Can you work these out from the model? Positions are in its coordinate system, mm. Face numbers are marked on the shaded views. A direction names the side the tool comes from. Coordinates: 2 decimals unless noted, no trailing zeros. Order: outer loops, then holes, each group sorted by start corner. A loop starts at its lowest first (then second) coordinate and runs counter-clockwise, first axis right, second up. Notation, with made-up numbers: (79, 78) -> (94, 78) arc R31 cw to (94, 106) -> close; hole circle Ø2 at (-14, 52). An arc over 180 degrees is marked (long way). Return JSON: item names as keys, results as strings. Group by question number.
1) If I drill on probe 1 along Z at (x, y) = (0, -1); probe 2 along X at (y, z) = (0.75, 209.55); probe 3 along X at (y, z) = (-2, 209.55), over which ranges is the centre line in solid material (lowest first)? Write a range as from..to.
2) For pin 1 (5 mm diameter, centred on x = -0.5, z = 205, fed in from -Y); pin 2 (3 mm diameter, centred on x = -1, z = 211, fed in from -Y); pin 3 (5 mm diameter, centred on x = -18.5, y = -16, fed in from +Z); pin 4 (2 mm diameter, centred on x = -44.5, y = -47.5, fed in from -Z), each with a flat end and sliding along its axis, tell me the tip position at first contact or that it passes through.
3) If we section it at A-A, the plane z = 161.5: Please give me the cut outline in (x, y), then the cut area to 3 significant figures.
4) For the marked faces 1 and 2, which set-ups out of +Z, -Z, +X, -X, +Y, -Y let a thin tool reach every point of the face, with its end or its side?
from build123d import *

# Parameters (mm, degrees)
F0_R      = 69.85
F1_DEPTH  = 12.7
F4_R      = 5.08
F5_R      = 6.35
F6_DEPTH  = 203.2
F8_DEPTH  = 12.7
F9_R      = 3.81
F10_DEPTH = 12.7
F11_R     = 5.08


with BuildPart() as f1:
    # F0 (on Top) → F1 (new body)
    with BuildSketch(Plane.XY):
        Circle(F0_R)
    extrude(amount=F1_DEPTH)

    # F2 (on Front) → F3 (revolve)
    with BuildSketch(Plane.XZ):
        Polygon((0, 50.8), (-69.85, 12.7), (0, 12.7), align=None)
    revolve(axis=Axis((0, 0, 31.75), (0, 0, -1)))

    # F4
    f4_edges = [f1.edges().sort_by_distance(p)[0] for p in [
        (0, -69.85, 12.7),
        (0, 69.85, 12.7),
    ]]
    fillet(f4_edges, radius=F4_R)

    # F5 (on Top) → F6 (join)
    with BuildSketch(Plane.XY):
        Circle(F5_R)
    extrude(amount=F6_DEPTH)

    # F7 (on face) → F8 (join)
    with BuildSketch(Plane.XY.offset(203.2)):
        with BuildLine():
            ThreePointArc((-3.81, 5.08), (-6.35, 0), (-3.81, -5.08))
            Line((-3.81, -5.08), (3.81, -5.08))
            ThreePointArc((3.81, -5.08), (6.35, 0), (3.81, 5.08))
            Line((3.81, 5.08), (-3.81, 5.08))
        make_face()
    extrude(amount=F8_DEPTH)

    # F9 (on face) → F10 (cut, symmetric)
    with BuildSketch(Plane.XZ.offset(5.08)):
        with Locations((0, 209.55)):
            Circle(F9_R)
    extrude(amount=F10_DEPTH, both=True, mode=Mode.SUBTRACT)

    # F11
    f11_edges = [f1.edges().sort_by_distance(p)[0] for p in [
        (0, -6.35, 47.336364),
        (0, 6.35, 47.336364),
        (-36.776284, 0, 30.740209),
        (3.3e-05, 67.202608, 14.144033),
        (3.3e-05, -67.202608, 14.144033),
    ]]
    fillet(f11_edges, radius=F11_R)


solid = f1.part
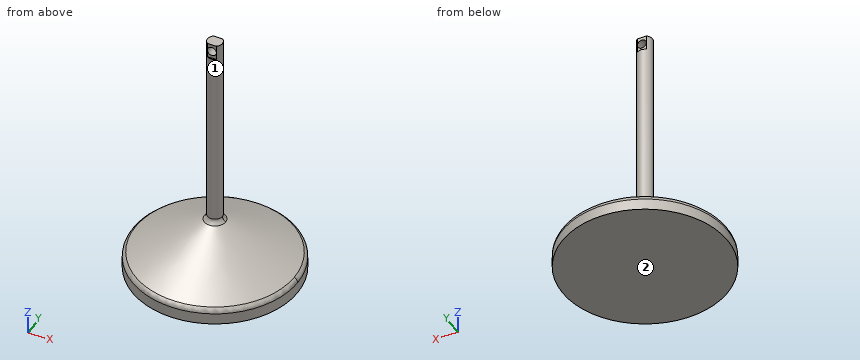
Result sheet:
{
 "1": {"probe 1": "z = 0..205.74, 213.36..215.9", "probe 2": "x = -6.31..-3.81, 3.81..6.31", "probe 3": "x = -6.03..-3.81, 3.81..6.03"},
 "2": {"pin 1": "stops at y = -6.35", "pin 2": "passes through", "pin 3": "stops at z = 38.82", "pin 4": "stops at z = 0"},
 "3": {"outline": "circle Ø12.7 at (0, 0)", "area": "127 mm2"},
 "4": {"face 1": "+Z", "face 2": "-Z, +X, -X, +Y, -Y"}
}
